Check sheet for the drawn part. Datum: minimum x, y, z corner. Units: mm. Round coordinates to 2 decimals unless told otherwise and drop trailing zeros. Order: outer loops, then holes, each group sorted by start corner. A loop starts at its lowest first (then second) coordinate and runs counter-clockwise, first axis right, second up. Notation, with made-up numbers: (83, 45) -> (102, 45) arc R25 cw to (102, 57) -> close; hole circle Ø10 at (-33.75, 20). An arc over 180 degrees is marked (long way). Answer as CSV lines item,"result". Start each with the question number.
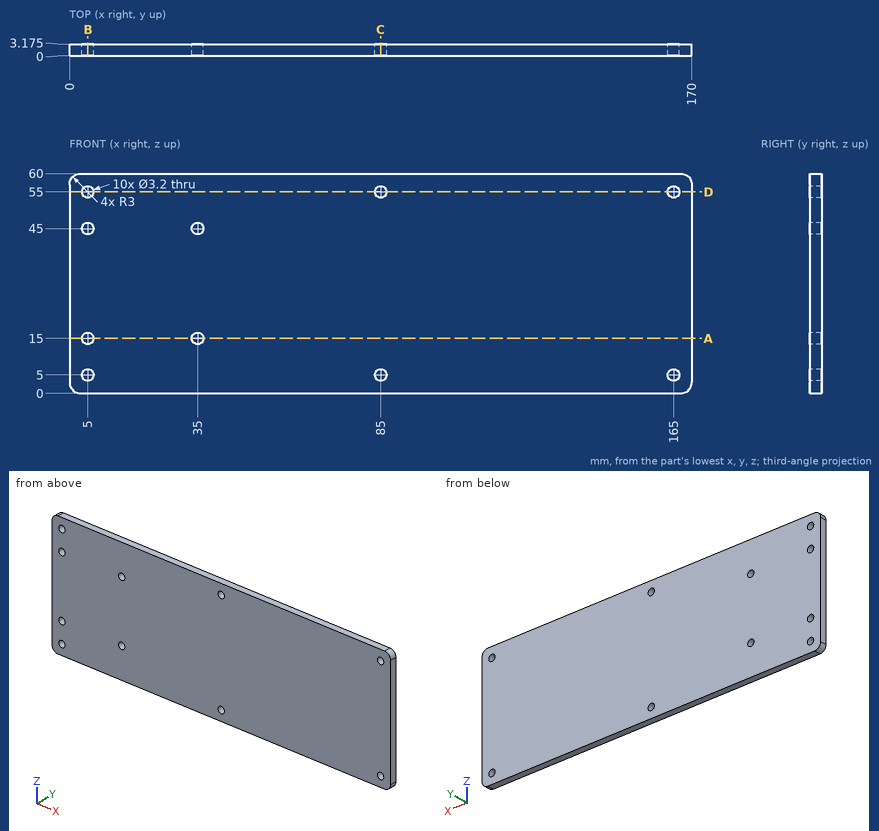
1) Section check A-A on z = 15. Record the cut outline in (x, y) (3 decimals), then the cut area to 3 significant figures.
2) Depth check by flat-ended pin: pin 1 Ø4 at (x, z) = (5, 15) entering from +Y (3 decimals); pin 2 Ø1.9 at (x, z) = (5, 5) entering from -Y. Enter the tip coordinate at first touch or a pass-through.
3) Material ranges on line 1 along Z through (x, y) = (35, 1.05); line 2 along Z through (x, y) = (5, 2.3); line 3 along X through (y, z) = (1.8, 15), recorded low to high.
4) Section check C-C on x = 85. Record the cut outline in (y, z) (3 decimals).
5) Section check B-B on x = 5. Record the cut outline in (y, z) (3 decimals), then the cut area to 3 significant figures.
6) Section check D-D on z = 55. Record the cut outline in (x, y) (3 decimals).
Solutions:
1,outline,"(0, 0) -> (3.4, 0) -> (3.4, 3.175) -> (0, 3.175) -> close; (6.6, 0) -> (33.4, 0) -> (33.4, 3.175) -> (6.6, 3.175) -> close; (36.6, 0) -> (170, 0) -> (170, 3.175) -> (36.6, 3.175) -> close"
1,area,"519 mm^2"
2,pin 1,"stops at y = 3.175"
2,pin 2,"passes through"
3,line 1,"z = 0 to 13.4, 16.6 to 43.4, 46.6 to 60"
3,line 2,"z = 0 to 3.4, 6.6 to 13.4, 16.6 to 43.4, 46.6 to 53.4, 56.6 to 60"
3,line 3,"x = 0 to 3.4, 6.6 to 33.4, 36.6 to 170"
4,outline,"(0, 0) -> (3.175, 0) -> (3.175, 3.4) -> (0, 3.4) -> close; (0, 6.6) -> (3.175, 6.6) -> (3.175, 53.4) -> (0, 53.4) -> close; (0, 56.6) -> (3.175, 56.6) -> (3.175, 60) -> (0, 60) -> close"
5,outline,"(0, 0) -> (3.175, 0) -> (3.175, 3.4) -> (0, 3.4) -> close; (0, 6.6) -> (3.175, 6.6) -> (3.175, 13.4) -> (0, 13.4) -> close; (0, 16.6) -> (3.175, 16.6) -> (3.175, 43.4) -> (0, 43.4) -> close; (0, 46.6) -> (3.175, 46.6) -> (3.175, 53.4) -> (0, 53.4) -> close; (0, 56.6) -> (3.175, 56.6) -> (3.175, 60) -> (0, 60) -> close"
5,area,"150 mm^2"
6,outline,"(0, 0) -> (3.4, 0) -> (3.4, 3.175) -> (0, 3.175) -> close; (6.6, 0) -> (83.4, 0) -> (83.4, 3.175) -> (6.6, 3.175) -> close; (86.6, 0) -> (163.4, 0) -> (163.4, 3.175) -> (86.6, 3.175) -> close; (166.6, 0) -> (170, 0) -> (170, 3.175) -> (166.6, 3.175) -> close"
